Print and shaded views of the part. All mm, measured from the part's lowest x, y and z. Round coordinates to 2 decimals unless told otherwise and drop trailing zeros. Order: outer loops, then holes, each group sorted by start corner. A loop starts at its lowest first (then second) coordinate and runs counter-clockwise, first axis right, second up. Notation, with made-up numbers: M 25.25,56.25 L 60.25,56.25 A13 ccw 60.25,77.25 Z; hole C 33.5,10.5 d1. An arc over 180 degrees is marked long. Write each question's results on one line, items separated by ' | '. Start each with the question number.
1. Drop flat-ended pins along their axis: pin 1 Ø6 at (y, z) = (4, 4) entering from -X; pin 2 Ø1 at (y, z) = (5.5, 24) entering from -X; pin 3 Ø7 at (x, y) = (8, 8) entering from +Z; pin 4 Ø3 at (y, z) = (4, 28.5) entering from +X. Give the stop position or say it passes through.
2. Probe L1, parallel to X at y = 8, z = 24.5; L2, parallel to X at y = 5.75, z = 9.5; L3, parallel to Y at x = 6.75, z = 9. List the from-to ranges inside material, lowest first. Write a range as [from, to].
3. Two-plate mould, pull along Y, no slides. Class the marked faces 1 and 2: +Y half, -Y half, draft (parallel to the pull), parting line (faces both ways), or undercut.
4. Band-saw the part on C-C, the plane z = 8.5. List the corners of the cut face in (x, y).
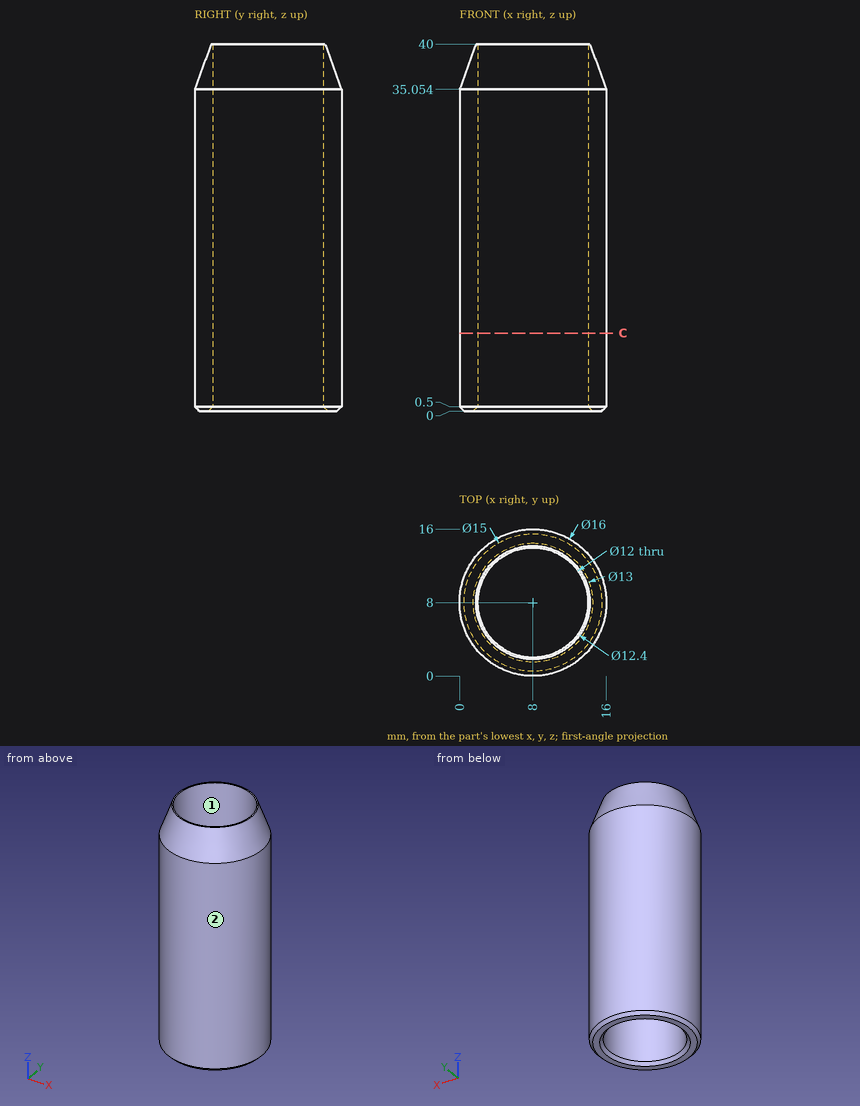
Solution:
1) pin 1: x = 0.06 | pin 2: x = 0.25 | pin 3: through | pin 4: x = 15.6
2) L1: [0, 2], [14, 16] | L2: [0.32, 2.44], [13.56, 15.68] | L3: [0.1, 2.13], [13.87, 15.9]
3) face 1: undercut | face 2: parting line
4) outline: C 8,8 d16; hole C 8,8 d12
